Build history of the part. All positions in model axes, mm. Face numbers are marked on the shaded views. A direction names the side the tool comes from. Round coordinates to 2 decimals unless told otherwise and drop trailing zeros. Loops run counter-clockwise (first coordinate to the right, second up) from the corner with the lowest first, then second, coordinate; pieces in that order, holes last. Notation, with made-up numbers: (61.25, 45) - (98.25, 45) arc R21 cw to (98.25, 83) - close; hole circle Ø11 at (-14, 0.5). An arc over 180 degrees is marked (long way). Use one line per item in the form item = value. Start each with the question number.
Q1. Saw through at D-D (y = -8). Give the cut face in (x, z), then the cut area to 3 significant figures.
Q2. Mould opens along Y. For the marked faces 1, 2 and 3 say: released by +Y, released by -Y, zero draft, split by the parting line, or undercut.
Q3. Saw through at C-C (x = 0.5). Give the cut face in (y, z).
Q4. Saw through at A-A (y = 0). Give the cut face in (x, z).
Q5. Drill centre lines: line 1 (Z direction, x = -4.25, y = 0); line 2 (Z direction, x = 2.75, y = 8.75); line 3 (X direction, y = 0.25, z = 4). Where is each one in solid material? Low to high.
Q6. 3-axis set-ups, long thin cutter, end or side, ignore diameter. For the marked faces 4, 5 and 6: which of +Z, -Z, +X, -X, +Y, -Y reach the whole face in a straight line?
Q7. Pin check, flat tips, straight feed: pin 1 (2.5 mm diameter, centred on y = 4, z = 11, fed in from -X); pin 2 (6 mm diameter, centred on y = -6.5, z = 4, fed in from -X); pin 3 (1.3 mm diameter, centred on y = -4, z = 10.5, fed in from +X). Stop position of each tip, or through.
Q8. Saw through at B-B (z = 4). Give the cut face in (x, y).
```python
from build123d import *

# Parameters (mm, degrees)
SKETCH_W        = 25
SKETCH_H        = 20
PAD_DEPTH       = 18
SKETCH001_R     = 1
POCKET_DEPTH    = 25.001
SKETCH002_W     = 6
SKETCH002_H     = 8
POCKET001_DEPTH = 20.001
SKETCH003_R     = 1.35
POCKET002_DEPTH = 15
CHAMFER_SIZE    = 8
CHAMFER001_SIZE = 2
SKETCH004_W     = 14.1
SKETCH004_H     = 13
POCKET003_DEPTH = 3
FILLET_R        = 0.5
CHAMFER002_SIZE = 7
FILLET001_R     = 1
POCKET004_DEPTH = 5
FILLET002_R     = 0.5
CHAMFER003_SIZE = 0.3


with BuildPart() as part:
    # Sketch (on XY_Plane of Origin) → Pad (new body)
    with BuildSketch(Plane.XY):
        Rectangle(SKETCH_W, SKETCH_H)
    extrude(amount=PAD_DEPTH)

    # Sketch001 (on Face4 of Pad) → Pocket (cut, through all)
    with BuildSketch(Plane(origin=(-12.5, 0, 0), x_dir=(0, -1, 0), z_dir=(-1, 0, 0))):
        with Locations((0, 14)):
            Circle(SKETCH001_R)
    extrude(amount=-POCKET_DEPTH, mode=Mode.SUBTRACT)

    # Sketch002 (on Face1 of Pocket) → Pocket001 (cut, through all)
    with BuildSketch(Plane.XZ.offset(10)):
        with Locations((9.5, 18)):
            Rectangle(SKETCH002_W, SKETCH002_H)
    extrude(amount=-POCKET001_DEPTH, mode=Mode.SUBTRACT)

    # Sketch003 (on Face3 of Pocket001) → Pocket002 (cut)
    with BuildSketch(Plane.YZ.offset(12.5)):
        with Locations((-4, 11)):
            Circle(SKETCH003_R)
    pocket002 = extrude(amount=-POCKET002_DEPTH, mode=Mode.SUBTRACT)

    # Mirrored: Pocket002 across XZ
    add(pocket002.mirror(Plane.XZ), mode=Mode.SUBTRACT)

    # Chamfer
    chamfer_edges = [part.edges().sort_by_distance(p)[0] for p in [
        (6.5, -10, 16),
        (6.5, 10, 16),
    ]]
    chamfer(chamfer_edges, length=CHAMFER_SIZE)

    # Chamfer001
    chamfer001_edges = [part.edges().sort_by_distance(p)[0] for p in [
        (6.5, 0, 18),
    ]]
    chamfer(chamfer001_edges, length=CHAMFER001_SIZE)

    # Sketch004 (on Face11 of Chamfer001) → Pocket003 (cut)
    with BuildSketch(Plane.YZ.offset(12.5)):
        with Locations((0, 8.5)):
            Rectangle(SKETCH004_W, SKETCH004_H)
    extrude(amount=-POCKET003_DEPTH, mode=Mode.SUBTRACT)

    # Fillet
    fillet_edges = [part.edges().sort_by_distance(p)[0] for p in [
        (12.5, -10, 7),
        (12.5, -7.05, 8),
        (12.5, 7.05, 8),
        (12.5, 10, 7),
    ]]
    fillet(fillet_edges, radius=FILLET_R)

    # Chamfer002
    chamfer002_edges = [part.edges().sort_by_distance(p)[0] for p in [
        (-12.5, -10, 9),
        (-12.5, 10, 9),
    ]]
    chamfer(chamfer002_edges, length=CHAMFER002_SIZE)

    # Fillet001
    fillet001_edges = [part.edges().sort_by_distance(p)[0] for p in [
        (-12.5, -3, 9),
        (-5.5, -10, 9),
        (-12.5, 3, 9),
        (-5.5, 10, 9),
    ]]
    fillet(fillet001_edges, radius=FILLET001_R)

    # Sketch005 (on Face2 of Fillet001) → Pocket004 (cut)
    with BuildSketch(Plane(origin=(0, 0, 0), x_dir=(1, 0, 0), z_dir=(0, 0, -1))):
        with BuildLine():
            ThreePointArc((11.5, 1.6), (9.9, 0), (11.5, -1.6))
            Line((11.5, -1.6), (21.5, -1.6))
            ThreePointArc((21.5, -1.6), (23.1, 0), (21.5, 1.6))
            Line((11.5, 1.6), (21.5, 1.6))
        make_face()
    extrude(amount=-POCKET004_DEPTH, mode=Mode.SUBTRACT)

    # Fillet002
    fillet002_edges = [part.edges().sort_by_distance(p)[0] for p in [
        (12.5, 1.6, 1),
        (12.5, -1.6, 1),
    ]]
    fillet(fillet002_edges, radius=FILLET002_R)

    # Chamfer003
    chamfer003_edges = [part.edges().sort_by_distance(p)[0] for p in [
        (3.457107, -10, 0),
    ]]
    chamfer(chamfer003_edges, length=CHAMFER003_SIZE)


solid = part.part
```
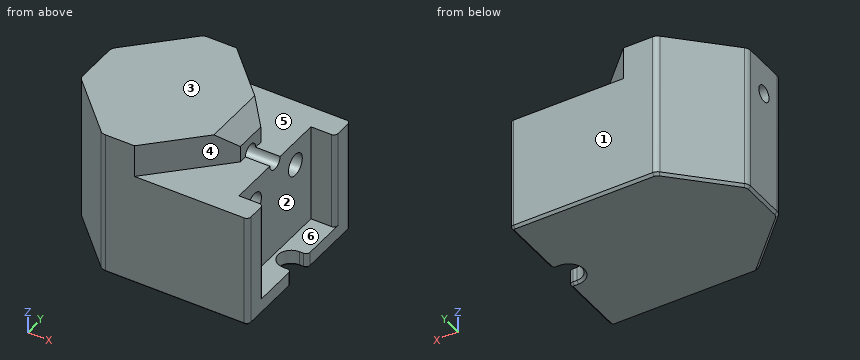
Report:
q1.outline = (-7.5, 0.3) - (-7.08, 0) - (12.2, 0) - (12.5, 0.3) - (12.5, 14) - (0.5, 14) - (0.5, 18) - (-7.5, 18) - close
q1.area = 312 mm²
q2.face_1 = released by +Y
q2.face_2 = undercut
q2.face_3 = zero draft
q3.outline = (-10, 0.3) - (-9.7, 0) - (9.7, 0) - (10, 0.3) - (10, 14) - (8, 14) - (8, 18) - (-8, 18) - (-8, 14) - (-10, 14) - close; hole circle Ø2.7 at (-4, 11); hole circle Ø2 at (0, 14); hole circle Ø2.7 at (4, 11)
q4.outline = (-12.5, 0.3) - (-12.2, 0) - (9.6, 0) - (9.9, 0.3) - (9.9, 2) - (9.5, 2) - (9.5, 13) - (-12.5, 13) - close; (-12.5, 15) - (6.5, 15) - (6.5, 16) - (4.5, 18) - (-12.5, 18) - close
q5.line_1 = 0 to 13, 15 to 18
q5.line_2 = 0 to 14
q5.line_3 = -12.5 to 9.5
q6.face_4 = +Z, +X, -Y
q6.face_5 = +Z, +X, +Y
q6.face_6 = +Z, +X
q7.pin_1 = -12.49
q7.pin_2 = -12
q7.pin_3 = -2.5
q8.outline = (-12.5, -2.59) arc R1 ccw to (-12.21, -3.29) - (-5.79, -9.71) arc R1 ccw to (-5.09, -10) - (12, -10) arc R0.5 ccw to (12.5, -9.5) - (12.5, -7.55) arc R0.5 ccw to (12, -7.05) - (9.5, -7.05) - (9.5, 7.05) - (12, 7.05) arc R0.5 ccw to (12.5, 7.55) - (12.5, 9.5) arc R0.5 ccw to (12, 10) - (-5.09, 10) arc R1 ccw to (-5.79, 9.71) - (-12.21, 3.29) arc R1 ccw to (-12.5, 2.59) - close
